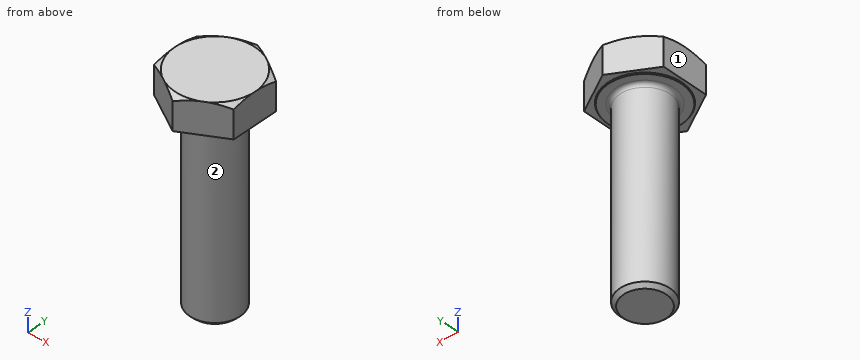
from build123d import *

# Parameters (mm, degrees)
BOSS_EXTRUDE1_DEPTH = 5.15


with BuildPart() as part:
    # Sketch1 → Boss-Extrude1 (new body)
    with BuildSketch(Plane.XY):
        Polygon((0, 7.349668927), (-6.365, 3.674834463), (-6.365, -3.674834463), (0, -7.349668927), (6.365, -3.674834463), (6.365, 3.674834463), align=None)
    extrude(amount=BOSS_EXTRUDE1_DEPTH)

    # Sketch2 → Revolve1 (revolve)
    with BuildSketch(Plane(origin=(0, 0, 0), x_dir=(0, 0, -1), z_dir=(1, 0, 0)), mode=Mode.PRIVATE) as revolve1_sk:
        with BuildLine():
            Line((0, 0), (0, 4.6))
            ThreePointArc((0, 4.6), (0.175735931, 4.175735931), (0.6, 4))
            Line((0.6, 4), (29.4, 4))
            Line((29.4, 4), (30, 3.4))
            Line((30, 3.4), (30, 0))
            Line((30, 0), (0, 0))
        make_face()
    revolve(revolve1_sk.sketch.rotate(Axis((0, 0, 0), (0, 0, -1)), 90), axis=Axis((0, 0, 0), (0, 0, -1)))

    # Sketch3 → Cut-Revolve1 (revolve, cut)
    with BuildSketch(Plane(origin=(0, 0, 0), x_dir=(0, 0, -1), z_dir=(1, 0, 0)), mode=Mode.PRIVATE) as cut_revolve1_sk:
        Polygon((-5.15, 7.349668927), (-4.58150113, 7.349668927), (-5.15, 6.365), align=None)
        Polygon((-0.15, 7.349668927), (-0.15, 5.88660254), (0, 5.8), (0, 7.349668927), align=None)
    revolve(cut_revolve1_sk.sketch.rotate(Axis((0, 0, 12.204941078), (0, 0, -1)), 90), axis=Axis((0, 0, 12.204941078), (0, 0, -1)), mode=Mode.SUBTRACT)


solid = part.part
Could you check a few things on this model? Use its own coordinates, in mm. Face numbers are marked on the shaded views. A direction names the side the tool comes from. Round coordinates to 2 decimals unless told otherwise and drop trailing zeros. Write each loop counter-clockwise with the first axis right and the second up, starting at its lowest first coordinate (ties: lowest second). Pieces come first, ordered by that corner, then holes. Notation, with made-up numbers: (-39, 83) - (-12, 83) arc R14 ccw to (-12, 108) - close; hole circle Ø7 at (32.5, 85). An arc over 180 degrees is marked (long way). Use a Markdown table: item, result.
Q1. For the marked faces 1 and 2, which set-ups out of +Z, -Z, +X, -X, +Y, -Y let a thin tool reach every point of the face, with its end or its side?
Output values:
| item | result |
|---|---|
| face 1 | +Z, -Z, -X, +Y, -Y |
| face 2 | -Z |
Q2. I want a section at A-A (z = -16.5). List the corners of the cut face in (x, y) for me.
Output values:
| item | result |
|---|---|
| outline | circle Ø8 at (0, 0) |
Q3. Please list where these lines run through material, in increasing order: L1, parallel to Y at x = -0.25, z = -24; L2, parallel to Z at x = 5.75, y = -1.75; L3, parallel to Z at x = 3.75, y = -3.5.
Output values:
| item | result |
|---|---|
| L1 | -3.99 to 3.99 |
| L2 | 0.15 to 5.15 |
| L3 | 0 to 5.15 |
Q4. For pin 1 (5 mm diameter, centred on x = 2.5, z = -21, fed in from +Y); pin 2 (5 mm diameter, centred on y = 1, z = -15.5, fed in from -X); pin 3 (5 mm diameter, centred on y = -3.5, z = -7.5, fed in from -X), each with a flat end and sliding along its axis, tell me the tip position at first contact or that it passes through.
Output values:
| item | result |
|---|---|
| pin 1 | y = 4 |
| pin 2 | x = -4 |
| pin 3 | x = -3.87 |
